```python
from build123d import *

# Parameters (mm, degrees)
F0_W           = 101.6
F0_H           = 101.6
F1_DEPTH       = 101.6
F2_R           = 25.4
F3_DEPTH       = 101.6
F4_R           = 25.4
F5_DEPTH       = 101.6
F6_R           = 25.4
F7_DEPTH       = 101.6
F8_R           = 6.35
F10_R          = 25.4
F11_DEPTH      = 50.8
F11_DEPTH_BACK = 152.4


with BuildPart() as f1:
    # F0 (on Front) → F1 (new body)
    with BuildSketch(Plane.XZ):
        with Locations((50.8, 50.8)):
            Rectangle(F0_W, F0_H)
    extrude(amount=F1_DEPTH)

    # F2 (on face) → F3 (cut)
    with BuildSketch(Plane.XY.offset(101.6)):
        with Locations((50.8, -50.8)):
            Circle(F2_R)
    extrude(amount=-F3_DEPTH, mode=Mode.SUBTRACT)

    # F4 (on face) → F5 (cut)
    with BuildSketch(Plane(origin=(0, 0, 0), x_dir=(0, -1, 0), z_dir=(-1, 0, 0))):
        with Locations((50.8, 50.8)):
            Circle(F4_R)
    extrude(amount=-F5_DEPTH, mode=Mode.SUBTRACT)

    # F6 (on face) → F7 (cut)
    with BuildSketch(Plane.XZ.offset(101.6)):
        with Locations((50.8, 50.8)):
            Circle(F6_R)
    extrude(amount=-F7_DEPTH, mode=Mode.SUBTRACT)

    # F8
    f8_edges = [f1.edges().sort_by_distance(p)[0] for p in [
        (0, -50.8, 101.6),
        (50.8, 0, 101.6),
        (101.6, -50.8, 101.6),
        (50.8, -101.6, 101.6),
        (0, -101.6, 50.8),
        (101.6, -101.6, 50.8),
        (101.6, 0, 50.8),
        (101.6, -50.8, 0),
        (50.8, -101.6, 0),
        (50.8, 0, 0),
        (0, 0, 50.8),
        (0, -50.8, 0),
    ]]
    fillet(f8_edges, radius=F8_R)

    # F10 (on offset) → F11 (join, two sides)
    with BuildSketch(Plane.XZ.offset(101.6)) as f11_sk:
        Circle(F10_R)
    extrude(amount=F11_DEPTH)
    extrude(f11_sk.sketch, amount=-F11_DEPTH_BACK)


solid = f1.part
```
Here's how the part is built. I have some questions about the finished solid (model axes, mm). A direction names the side the tool comes from. Coordinates: 2 decimals unless noted, no trailing zeros. Write each loop counter-clockwise with the first axis right and the second up, starting at its lowest first coordinate (ties: lowest second). Pieces come first, ordered by that corner, then holes. Notation, with made-up numbers: (61.25, 10) -> (92.25, 10) arc R14 ccw to (92.25, 14) -> close; hole circle Ø8 at (80.5, -3.5). An arc over 180 degrees is marked (long way). Use a Markdown table: item, result. Add a question column.
(1) I'm going to push flat-ended pins straight in: P1, Ø1, axis at x = -12.5, y = -73, coming from the -Z side; P2, Ø6, axis at y = -111, z = -11, coming from the -X side; P3, Ø8, axis at x = 6, y = -113.5, coming from the +Z side. Where does each tip first touch, or does it pass through?
(2) Please list where these lines run through material, in increasing order: line 1 (Z direction, x = 79, y = -50.8); line 2 (Y direction, x = 51, z = 9).
(3) For faces 5 (the flat face through (0, -60, 75)), 6 (the cylindrical face through (32.08, -33.63, 89.06)), 7 (the cylindrical face through (1.81, -1.91, 60.42)), which set-ups out of +Z, -Z, +X, -X, +Y, -Y let a thin tool reach every point of the face, with its end or its side?
(4) If we section it at D-D, the plane x = 10: Write out the boundary of the cut face in (y, z).
(5) If we section it at B-B, the plane x = 50.8: Write out the boundary of the cut face in (y, z), and give its area (3 significant figures).
(6) If we section it at A-A, the plane y = -89.5: Write out the boundary of the cut face in (x, z).
(7) If we section it at C-C, the plane z = 50.8: Write out the boundary of the cut face in (x, y).
(8) We'd pull the mould along Y, two halves only. Please class faces 1 (the cylindrical face through (60.42, -1.91, 1.81)), 2 (the cylindrical face through (88.6, -32.08, 67.97)), 3 (the cylindrical face through (99.69, -51.42, 99.79)), 4 (the cylindrical face through (51.42, -99.79, 99.69)): +Y half, -Y half, draft (parallel to the pull), parting line (faces both ways), or undercut.
Outcome:
| question | item | result |
|---|---|---|
| 1 | P1 | stops at z = -22.39 |
| 1 | P2 | stops at x = -24.11 |
| 1 | P3 | stops at z = 25.32 |
| 2 | line 1 | z = 0 to 25.4, 76.2 to 101.6 |
| 2 | line 2 | y = -101.6 to -76.2, -25.4 to 0 |
| 3 | face 5 | +Z, -X, +Y, -Y |
| 3 | face 6 | +Z, -Z |
| 3 | face 7 | +Z, -X, +Y |
| 4 | outline | (-152.4, -23.35) -> (50.8, -23.35) -> (50.8, 23.35) -> (0, 23.35) -> (0, 95.25) arc R6.35 ccw to (-6.35, 101.6) -> (-95.25, 101.6) arc R6.35 ccw to (-101.6, 95.25) -> (-101.6, 23.35) -> (-152.4, 23.35) -> close; hole circle Ø50.8 at (-50.8, 50.8) |
| 5 | outline | (-101.6, 6.35) arc R6.35 ccw to (-95.25, 0) -> (-76.2, 0) -> (-76.2, 25.4) -> (-101.6, 25.4) -> close; (-101.6, 76.2) -> (-76.2, 76.2) -> (-76.2, 101.6) -> (-95.25, 101.6) arc R6.35 ccw to (-101.6, 95.25) -> close; (-25.4, 0) -> (-6.35, 0) arc R6.35 ccw to (0, 6.35) -> (0, 25.4) -> (-25.4, 25.4) -> close; (-25.4, 76.2) -> (0, 76.2) -> (0, 95.25) arc R6.35 ccw to (-6.35, 101.6) -> (-25.4, 101.6) -> close |
| 5 | area | 2,550 mm^2 |
| 6 | outline | (0, 25.4) arc R25.4 ccw (long way) to (25.4, 0) -> (95.25, 0) arc R6.35 ccw to (101.6, 6.35) -> (101.6, 95.25) arc R6.35 ccw to (95.25, 101.6) -> (6.35, 101.6) arc R6.35 ccw to (0, 95.25) -> close; hole circle Ø50.8 at (50.8, 50.8) |
| 7 | outline | (0, -95.25) arc R6.35 ccw to (6.35, -101.6) -> (25.4, -101.6) -> (25.4, -76.2) -> (0, -76.2) -> close; (0, -25.4) -> (25.4, -25.4) -> (25.4, 0) -> (6.35, 0) arc R6.35 ccw to (0, -6.35) -> close; (76.2, -101.6) -> (95.25, -101.6) arc R6.35 ccw to (101.6, -95.25) -> (101.6, -76.2) -> (76.2, -76.2) -> close; (76.2, -25.4) -> (101.6, -25.4) -> (101.6, -6.35) arc R6.35 ccw to (95.25, 0) -> (76.2, 0) -> close |
| 8 | face 1 | +Y half |
| 8 | face 2 | undercut |
| 8 | face 3 | draft |
| 8 | face 4 | -Y half |
